Design review of the part built by this model. Coordinates are the model's own, in mm. Face numbers are marked on the shaded views. A direction names the side the tool comes from. Coordinates: 2 decimals unless noted, no trailing zeros. Loops run counter-clockwise (first coordinate to the right, second up) from the corner with the lowest first, then second, coordinate; pieces in that order, holes last. Notation, with made-up numbers: (23.5, 76.25) - (33.5, 76.25) arc R15 ccw to (33.5, 91.25) - close; hole circle Ø2 at (-16, 23.25). An arc over 180 degrees is marked (long way). Answer in a Markdown table with one row per item. Add a question column.
(1) We need section D-D, the plane x = -18. Write out the cut boundary in (y, z), plus the area to 3 significant figures.
(2) We need section A-A, the plane y = 231. Write out the cut boundary in (x, z).
(3) Clearance check with flat-ended pins moving along their axes: pin 1 (5 mm diameter, centred on y = 215.3, z = 28.9, fed in from +X); pin 2 (1.5 mm diameter, centred on x = -11, y = 117, fed in from +Z); pin 3 (6 mm diameter, centred on y = 95, z = 31, fed in from -X). State where each tip first meets the part, or that it passes through.
(4) We need section B-B, the plane z = 28.9. Write out the cut boundary in (x, y) (3 decimals).
(5) To check wall thickness, follow L1, parallel to Y at x = -31, z = 3; L2, parallel to Y at x = -5.5, z = 28.9 (3 decimals); L3, parallel to X at y = 60, z = 5. State the ranges of each line that lie inside material, in increasing order. Write a range as [from, to].
(6) For the marked faces 1 and 2, list the 3-axis set-ups (+Z, -Z, +X, -X, +Y, -Y) from which the entire face can be reached by the end or side of a thin tool; tool diameter is ignored.
(7) We need section C-C, the plane z = 41.5. Write out the cut boundary in (x, y).
Autodesk Inventor part; units mm, degrees
ref_plane "YZ Plane" through (0, 0, 0) normal (1, 0, 0) x (0, 1, 0)
ref_plane "XZ Plane" through (0, 0, 0) normal (0, 1, 0) x (-1, 0, 0)
ref_plane "XY Plane" through (0, 0, 0) normal (0, 0, 1) x (1, 0, 0)
sketch "Sketch1" plane through (0, 0, 0) normal (0, 1, 0) x (-1, 0, 0)
  line L0 (0, 0) -> (0, 49.7)
  line L1 (0, 49.7) -> (8, 49.7)
  line L2 (8, 49.7) -> (8, 8)
  line L3 (8, 8) -> (49.7, 8)
  line L4 (49.7, 8) -> (49.7, 0)
  line L5 (49.7, 0) -> (0, 0)
  dimension "d0" = 49.7
  dimension "d1" = 8
extrude "Extrusion1" add sketch "Sketch1" along normal blind 265
sketch "Sketch2" plane through (0, 0, 0) normal (0, 0, -1) x (-1, 0, 0)
  line L0 (49.7, 0) -> (0, 0) construction
  line L1 (49.7, 0) -> (49.7, 265) construction
  line L2 (0, 265) -> (49.7, 265) construction
  line L3 (0, 0) -> (0, 265) construction
  line L4 (31, 0) -> (31, 265) construction
  line L5 (0, 265) -> (49.7, 265) construction
  point P0 (31, 231)
  point P1 (31, 205)
  point P2 (31, 60)
  point P3 (31, 34)
  dimension "d4" = 26
  dimension "d5" = 26
  dimension "d6" = 34
  dimension "d7" = 34
  dimension "d8" = 31
hole "Hole1" at (-31, 231, 0) at (-31, 205, 0) at (-31, 60, 0) at (-31, 34, 0) direction (0, 0, 1) diameter 5.5 depth 8 tip angle 118
sketch "Sketch3" plane through (0, 0, 49.7) normal (1, 0, 0) x (0, 0, -1)
  line L0 (49.7, 0) -> (0, 0) construction
  line L1 (49.7, 0) -> (49.7, 265) construction
  line L2 (0, 265) -> (49.7, 265) construction
  line L3 (0, 0) -> (0, 265) construction
  line L4 (0, 0) -> (41.7, 0) construction
  line L5 (20.8, 0) -> (20.8, 265) construction
  point P0 (20.8, 132.5)
  point P1 (20.8, 215.3)
  point P2 (20.8, 49.7)
  dimension "d16" = 20.8
  dimension "Mounting_Hole_Spacing" = 82.8
  dimension "d18" = 82.8
hole "Hole2" at (0, 132.5, 28.9) at (0, 215.3, 28.9) at (0, 49.7, 28.9) direction (-1, 0, 0) diameter 8.45 end through all
properties part number "Horn_Bracket" material "Steel, Cast"
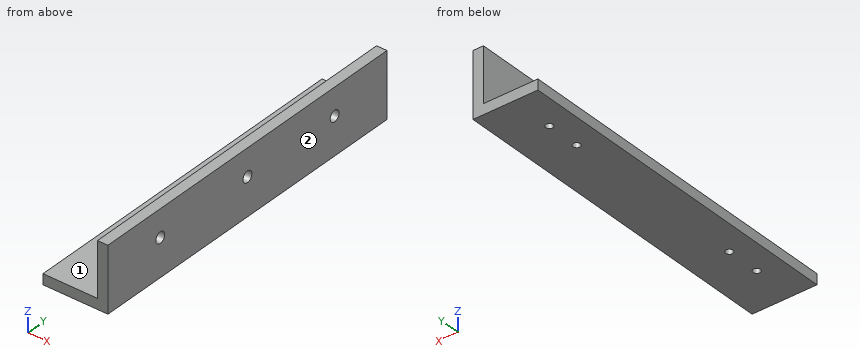
Responses:
| question | item | result |
|---|---|---|
| 1 | outline | (0, 0) - (265, 0) - (265, 8) - (0, 8) - close |
| 1 | area | 2,120 mm2 |
| 2 | outline | (-49.7, 0) - (-33.75, 0) - (-33.75, 8) - (-49.7, 8) - close; (-28.25, 0) - (0, 0) - (0, 49.7) - (-8, 49.7) - (-8, 8) - (-28.25, 8) - close |
| 3 | pin 1 | passes through |
| 3 | pin 2 | stops at z = 8 |
| 3 | pin 3 | stops at x = -8 |
| 4 | outline | (-8, 0) - (0, 0) - (0, 45.475) - (-8, 45.475) - close; (-8, 53.925) - (0, 53.925) - (0, 128.275) - (-8, 128.275) - close; (-8, 136.725) - (0, 136.725) - (0, 211.075) - (-8, 211.075) - close; (-8, 219.525) - (0, 219.525) - (0, 265) - (-8, 265) - close |
| 5 | L1 | y = [0, 31.25], [36.75, 57.25], [62.75, 202.25], [207.75, 228.25], [233.75, 265] |
| 5 | L2 | y = [0, 45.475], [53.925, 128.275], [136.725, 211.075], [219.525, 265] |
| 5 | L3 | x = [-49.7, -33.75], [-28.25, 0] |
| 6 | face 1 | +Z, -X, +Y, -Y |
| 6 | face 2 | +Z, -Z, +X, +Y, -Y |
| 7 | outline | (-8, 0) - (0, 0) - (0, 265) - (-8, 265) - close |
